```python
from build123d import *

# Parameters (mm, degrees)
F0_R     = 4
F1_DEPTH = 3
F2_R     = 6
F3_DEPTH = 2.5
F4_SIZE  = 1.99999
F5_R     = 4.5
F6_DEPTH = 1


# Not quite as in the source:
# - a fillet or chamfer that OpenCascade refuses, or shapes differently, is made with other operations: its cross-section is extruded or revolved along the edge and cut away or added
# - a fillet or chamfer is up to 0.001 mm smaller than in the source, because OpenCascade refuses the exact size


with BuildPart() as f1:
    # F0 (on Top) → F1 (new body)
    with BuildSketch(Plane.XY):
        Circle(F0_R)
    extrude(amount=F1_DEPTH)

    # F2 (on face) → F3 (join)
    with BuildSketch(Plane.XY.offset(3)):
        Circle(F2_R)
    extrude(amount=F3_DEPTH)

    # F4 (size 2 in the source; OpenCascade refuses exactly that, so slightly less here)
    f4_edges = [f1.edges().sort_by_distance(p)[0] for p in [
        (-6, 0, 3),
    ]]
    chamfer(f4_edges, length=F4_SIZE)

    # F5 (on face) → F6 (cut)
    with BuildSketch(Plane.XY.offset(5.5)):
        Circle(F5_R)
    extrude(amount=-F6_DEPTH, mode=Mode.SUBTRACT)

    # F7: fillet of radius 5 on 1 edges, made by hand

    # F7_s1 → F7_t2 (revolve)
    with BuildSketch(Plane.XZ):
        with BuildLine():
            ThreePointArc((4.5, 5.5), (3.0811388301, 4.7565835097), (1.5, 4.5))
            Line((1.5, 4.5), (4.5, 4.5))
            Line((4.5, 4.5), (4.5, 5.5))
        make_face()
    revolve(axis=Axis((0, 0, 4.5), (0, 0, 1)))


solid = f1.part
```
Design review of the part built by this model. Coordinates are the model's own, in mm. Round coordinates to 2 decimals unless told otherwise and drop trailing zeros. Write each loop counter-clockwise with the first axis right and the second up, starting at its lowest first coordinate (ties: lowest second). Pieces come first, ordered by that corner, then holes. Notation, with made-up numbers: (81, -28) -> (130, -28) arc R11 ccw to (130, -22) -> close; hole circle Ø11 at (81.5, 2.5). An arc over 180 degrees is marked (long way). Write item = value, one per line. Start each with the question number.
1) Take a section at B-B, the plane z = 4.3. State the section outline as (x, y) points.
2) Take a section at A-A, the plane z = 2.65. State the section outline as (x, y) points, plus the area to 3 significant figures.
3) Clearance check with flat-ended pins moving along their axes: pin 1 (2 mm diameter, centred on x = 2, z = 2.5, fed in from +Y); pin 2 (1.5 mm diameter, centred on x = 2, z = 5, fed in from +Y); pin 3 (3 mm diameter, centred on x = 3, z = 2, fed in from +Y). State where each tip first meets the part, or that it passes through.
4) Mouldability with a two-part tool opening along Y and no side actions: class faces 1 (the face through (-1.4, 4.5, 5.5)), 2 (the face through (-0.867, -3.905, 1.479)), 3 (the face through (0, 0, 4.5)) as +Y half, -Y half, draft (parallel to the pull), parting line (faces both ways), or undercut.
5) Wall thickness on probe 1 along Z at (x, y) = (-5.5, -1.5); probe 2 along Z at (x, y) = (0.75, 0.25); probe 3 along X at (y, z) = (-2, 5.2): over which ranges is each line inside the solid? List them lowest first. Write a range as from..to.
Results list:
q1.outline = circle Ø10.6 at (0, 0)
q2.outline = circle Ø8 at (0, 0)
q2.area = 50.3 mm²
q3.pin_1 = 4.12
q3.pin_2 = 5.87
q3.pin_3 = 3.71
q4.face_1 = draft
q4.face_2 = parting line
q4.face_3 = undercut
q5.probe_1 = 4.7..5.5
q5.probe_2 = 0..4.5
q5.probe_3 = -5.66..-3.52, 3.52..5.66
